from build123d import *

# Parameters (mm, degrees)
SKETCH_R    = 4.5
SKETCH_R_2  = 12
SKETCH_R_3  = 3
SKETCH_R_4  = 2.5
PAD_DEPTH   = 10
FILLET_R    = 10
FILLET001_R = 1


with BuildPart() as part:
    # Sketch → Pad (new body)
    with BuildSketch(Plane.XY):
        Polygon((-25, 45), (55, 45), (55, -75), (35, -75), (35, -115), (-25, -115), align=None)
        Circle(SKETCH_R, mode=Mode.SUBTRACT)
        with Locations((0, -85)):
            Circle(SKETCH_R_2, mode=Mode.SUBTRACT)
        with Locations((-10, -52)):
            Circle(SKETCH_R_3, mode=Mode.SUBTRACT)
        with Locations((40, -52)):
            Circle(SKETCH_R_3, mode=Mode.SUBTRACT)
        with Locations((40, 22)):
            Circle(SKETCH_R_3, mode=Mode.SUBTRACT)
        with Locations((-10, 22)):
            Circle(SKETCH_R_3, mode=Mode.SUBTRACT)
        with Locations((25, -80)):
            Circle(SKETCH_R_4, mode=Mode.SUBTRACT)
        with Locations((-18, -80)):
            Circle(SKETCH_R_4, mode=Mode.SUBTRACT)
    extrude(amount=PAD_DEPTH)

    # Fillet
    fillet_edges = [part.edges().sort_by_distance(p)[0] for p in [
        (35, -115, 5),
        (-25, -115, 5),
        (35, -75, 5),
        (-25, 45, 5),
    ]]
    fillet(fillet_edges, radius=FILLET_R)

    # Fillet001
    fillet001_edges = [part.edges().sort_by_distance(p)[0] for p in [
        (55, -75, 5),
        (55, 45, 5),
    ]]
    fillet(fillet001_edges, radius=FILLET001_R)


solid = part.part
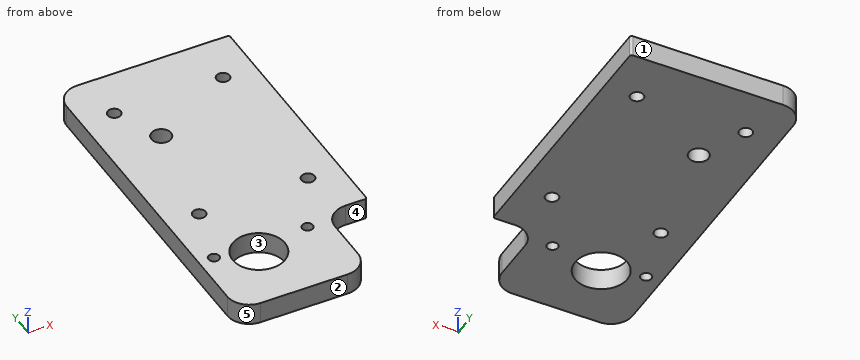
Model file for the job. Use its own axes, mm. Face numbers are marked on the shaded views. A direction names the side the tool comes from. Round coordinates to 2 decimals unless told otherwise and drop trailing zeros. Order: outer loops, then holes, each group sorted by start corner. A loop starts at its lowest first (then second) coordinate and runs counter-clockwise, first axis right, second up. Notation, with made-up numbers: M 19.5,4.5 L 68.5,4.5 A20 cw 68.5,10.5 Z; hole C 19.25,75 d8. An arc over 180 degrees is marked long. Write each question's results on one line, items separated by ' | '. Start each with the question number.
(1) Saw through at A-A, the plane y = 0. Give the cut face in (x, z).
(2) Drop flat-ended pins along their axis: pin 1 (2.5 mm diameter, centred on x = 47.5, z = 6.5, fed in from -Y); pin 2 (3 mm diameter, centred on x = 28.5, z = 6.5, fed in from -Y); pin 3 (5 mm diameter, centred on y = -99.5, z = 3, fed in from +X). Give the stop position or say it passes through.
(3) Two-plate mould, pull along Y, no slides. Class the marked faces 1, 2 and 3: pulls with the +Y half, pulls with the -Y half, needs draft (parallel to the pull), parting line crosses it, or undercut.
(4) Saw through at B-B, the plane x = 0. Give the cut face in (y, z).
(5) Saw through at D-D, the plane z = 3. State how many separate pieces and enclosed holes the cut face has, then the cut area to 3 significant figures.
(6) Probe probe 1 along Y at (x, z) = (0, 4.5); probe 2 along Y at (x, z) = (-10, 3.75); probe 3 along Y at (x, z) = (25, 2.5). List the from-to ranges inside material, lowest first. Write a range as from..to.
(7) Which spindle directions (+Z, -Z, +X, -X, +Y, -Y) get a long thin tool onto all of the face, cutting with end or side? Do the marked faces 4 and 5. Say none if no direction does.
(8) Saw through at C-C, the plane y = -52. Give the cut face in (x, z), then the cut area to 3 significant figures.
Established:
1) outline: M -25,0 L -4.5,0 L -4.5,10 L -25,10 Z; M 4.5,0 L 55,0 L 55,10 L 4.5,10 Z
2) pin 1: stops at y = -75 | pin 2: stops at y = -114.8 | pin 3: stops at x = 35
3) face 1: pulls with the +Y half | face 2: pulls with the -Y half | face 3: undercut
4) outline: M -115,0 L -97,0 L -97,10 L -115,10 Z; M -73,0 L -4.5,0 L -4.5,10 L -73,10 Z; M 4.5,0 L 45,0 L 45,10 L 4.5,10 Z
5) separate pieces: 1 | enclosed holes: 8 | area: 11,300 mm^2
6) probe 1: y = -115..-97, -73..-4.5, 4.5..45 | probe 2: y = -115..-91.63, -78.37..-55, -49..19, 25..45 | probe 3: y = -115..-82.5, -77.5..45
7) face 4: +Z, -Z, +X, -Y | face 5: +Z, -Z, -X, -Y
8) outline: M -25,0 L -13,0 L -13,10 L -25,10 Z; M -7,0 L 37,0 L 37,10 L -7,10 Z; M 43,0 L 55,0 L 55,10 L 43,10 Z | area: 680 mm^2
